Here's how the part is built. I have some questions about the finished solid (model axes, mm). Give positions to 0.01 mm unless a question says otherwise; leave off trailing zeros. Write each loop counter-clockwise with the first axis right and the second up, starting at its lowest first coordinate (ties: lowest second). Pieces come first, ordered by that corner, then holes. Notation, with made-up numbers: (75.5, 16.25) - (79.5, 16.25) arc R32 ccw to (79.5, 48.25) - close; hole circle Ø10 at (-33.75, 89). An arc over 180 degrees is marked (long way). One line per item, written item: value. Start each with the question number.
1) Imagine slicing it at D-D on x = -6. Write out the boundary of the cut face in (y, z) (3 decimals), plus the area to 3 significant figures.
2) Imagine slicing it at B-B on y = 0.5. Write out the boundary of the cut face in (x, z) (3 decimals).
3) Imagine slicing it at A-A on x = 1.75. Write out the boundary of the cut face in (y, z) (3 decimals), plus the area to 3 significant figures.
4) Please list where these lines run through material, in increasing order: L1, parallel to X at y = 0.45, z = -4.5 (3 decimals); L2, parallel to Z at x = 2.5, y = 0.1 (3 decimals); L3, parallel to X at y = 0.3, z = 5.5 (3 decimals). Write a range as [from, to].
5) Imagine slicing it at C-C on x = -0.75. Count the separate pieces of the cut face and the enclosed holes in it, plus the area to 3 significant figures.
from build123d import *

# Parameters (mm, degrees)
BOSS_EXTRUDE1_DEPTH     = 0.6
CUT_EXTRUDE1_DEPTH      = 14.483740208
CUT_EXTRUDE1_DEPTH_BACK = 14.483740208
CUT_EXTRUDE2_REACH      = 15.484


with BuildPart() as part:
    # Sketch1 → Boss-Extrude1 (new body)
    with BuildSketch(Plane(origin=(0, 0, 0), x_dir=(1, 0, 0), z_dir=(0, 1, 0))):
        with BuildLine():
            Line((-5.125, -7.025), (-5.125, -9.098312567))
            ThreePointArc((-5.125, -9.098312567), (-7.344632392, -8.642138452), (-9.525, -8.025))
            Line((-9.525, -8.025), (-9.525, 9.525))
            Line((-9.525, 9.525), (9.525, 9.525))
            Line((9.525, 9.525), (9.525, -8.025))
            ThreePointArc((9.525, -8.025), (7.344632392, -8.642138452), (5.125, -9.098312567))
            Line((5.125, -9.098312567), (5.125, -7.025))
            ThreePointArc((5.125, -7.025), (3.25, -5.15), (1.375, -7.025))
            Line((1.375, -7.025), (1.375, -9.494483029))
            ThreePointArc((1.375, -9.494483029), (0, -9.525), (-1.375, -9.494483029))
            Line((-1.375, -9.494483029), (-1.375, -7.025))
            ThreePointArc((-1.375, -7.025), (-3.25, -5.15), (-5.125, -7.025))
        make_face()
    extrude(amount=BOSS_EXTRUDE1_DEPTH)

    # Sketch2 → Cut-Extrude1 (cut, two sides: drawn at the far end of the back side and taken through both)
    with BuildSketch(Plane(origin=(0, 0, 0), x_dir=(0, 0, -1), z_dir=(1, 0, 0)).offset(-CUT_EXTRUDE1_DEPTH_BACK)):
        Polygon((-9.525, 0), (-8.025, 0.6), (-9.525, 0.6), align=None)
    extrude(amount=CUT_EXTRUDE1_DEPTH + CUT_EXTRUDE1_DEPTH_BACK, mode=Mode.SUBTRACT)

    # Sketch3 → Cut-Extrude2 (cut, up to next)
    with BuildSketch(Plane(origin=(0, 0.6, 0), x_dir=(1, 0, 0), z_dir=(0, 1, 0)), mode=Mode.PRIVATE) as cut_extrude2_sk1:
        with BuildLine():
            Line((2.5992936, 6.713604042), (-2.5992936, 6.713604042))
            ThreePointArc((-2.5992936, 6.713604042), (-3.297389596, 7.411700037), (-2.5992936, 8.109796033))
            Line((-2.5992936, 8.109796033), (2.5992936, 8.109796033))
            ThreePointArc((2.5992936, 8.109796033), (3.297389596, 7.411700037), (2.5992936, 6.713604042))
        make_face()
    cut_extrude2_tool1 = extrude(cut_extrude2_sk1.sketch, amount=-CUT_EXTRUDE2_REACH, mode=Mode.PRIVATE) & part.part
    # Sketch3 → Cut-Extrude2 (cut, up to next)
    with BuildSketch(Plane(origin=(0, 0.6, 0), x_dir=(1, 0, 0), z_dir=(0, 1, 0)), mode=Mode.PRIVATE) as cut_extrude2_sk2:
        with BuildLine():
            Line((2.5992936, 3.713604042), (-2.5992936, 3.713604042))
            ThreePointArc((-2.5992936, 3.713604042), (-3.297389596, 4.411700037), (-2.5992936, 5.109796033))
            Line((-2.5992936, 5.109796033), (2.5992936, 5.109796033))
            ThreePointArc((2.5992936, 5.109796033), (3.297389596, 4.411700037), (2.5992936, 3.713604042))
        make_face()
    cut_extrude2_tool2 = extrude(cut_extrude2_sk2.sketch, amount=-CUT_EXTRUDE2_REACH, mode=Mode.PRIVATE) & part.part
    # Sketch3 → Cut-Extrude2 (cut, up to next)
    with BuildSketch(Plane(origin=(0, 0.6, 0), x_dir=(1, 0, 0), z_dir=(0, 1, 0)), mode=Mode.PRIVATE) as cut_extrude2_sk3:
        with BuildLine():
            Line((2.5992936, 0.713604042), (-2.5992936, 0.713604042))
            ThreePointArc((-2.5992936, 0.713604042), (-3.297389596, 1.411700037), (-2.5992936, 2.109796033))
            Line((-2.5992936, 2.109796033), (2.5992936, 2.109796033))
            ThreePointArc((2.5992936, 2.109796033), (3.297389596, 1.411700037), (2.5992936, 0.713604042))
        make_face()
    cut_extrude2_tool3 = extrude(cut_extrude2_sk3.sketch, amount=-CUT_EXTRUDE2_REACH, mode=Mode.PRIVATE) & part.part
    add(cut_extrude2_tool1.solids().sort_by_distance((0, 0.6, -7.4117))[0], mode=Mode.SUBTRACT)
    add(cut_extrude2_tool2.solids().sort_by_distance((0, 0.6, -4.4117))[0], mode=Mode.SUBTRACT)
    add(cut_extrude2_tool3.solids().sort_by_distance((0, 0.6, -1.4117))[0], mode=Mode.SUBTRACT)


solid = part.part
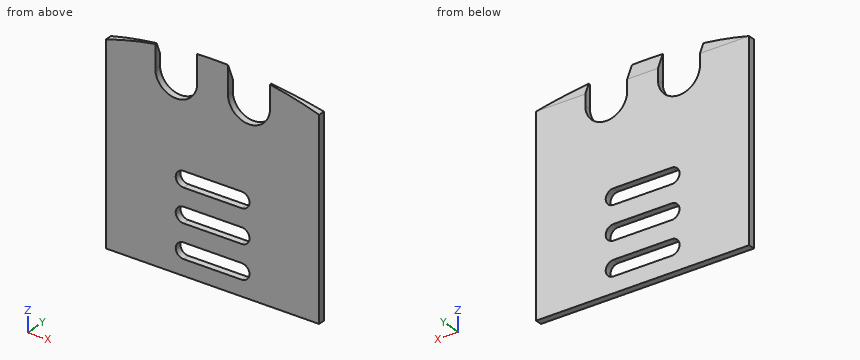
Numbers:
1. outline: (0, -9.525) - (0.6, -9.525) - (0.6, 8.025) - (0.235, 8.939) - (0, 8.939) - close
1. area: 10.9 mm^2
2. outline: (-9.525, -9.525) - (9.525, -9.525) - (9.525, 8.025) arc R30.992 ccw to (8.713, 8.275) - (5.125, 8.275) - (5.125, 7.025) arc R1.875 cw to (1.375, 7.025) - (1.375, 8.275) - (-1.375, 8.275) - (-1.375, 7.025) arc R1.875 cw to (-5.125, 7.025) - (-5.125, 8.275) - (-8.713, 8.275) arc R30.992 ccw to (-9.525, 8.025) - close; hole (-2.599, -8.11) - (2.599, -8.11) arc R0.698 ccw to (2.599, -6.714) - (-2.599, -6.714) arc R0.698 ccw to start; hole (-2.599, -5.11) - (2.599, -5.11) arc R0.698 ccw to (2.599, -3.714) - (-2.599, -3.714) arc R0.698 ccw to start; hole (-2.599, -2.11) - (2.599, -2.11) arc R0.698 ccw to (2.599, -0.714) - (-2.599, -0.714) arc R0.698 ccw to start
3. outline: (0, -9.525) - (0.6, -9.525) - (0.6, -8.11) - (0, -8.11) - close; (0, -6.714) - (0.6, -6.714) - (0.6, -5.11) - (0, -5.11) - close; (0, -3.714) - (0.6, -3.714) - (0.6, -2.11) - (0, -2.11) - close; (0, -0.714) - (0.6, -0.714) - (0.6, 5.9) - (0, 5.9) - close
3. area: 6.74 mm^2
4. L1: [-9.525, -3.292], [3.292, 9.525]
4. L2: [-9.525, -8.11], [-6.714, -5.11], [-3.714, -2.11], [-0.714, 5.307]
4. L3: [-9.525, -4.341], [-2.159, 2.159], [4.341, 9.525]
5. separate pieces: 4
5. enclosed holes: 0
5. area: 8.47 mm^2
